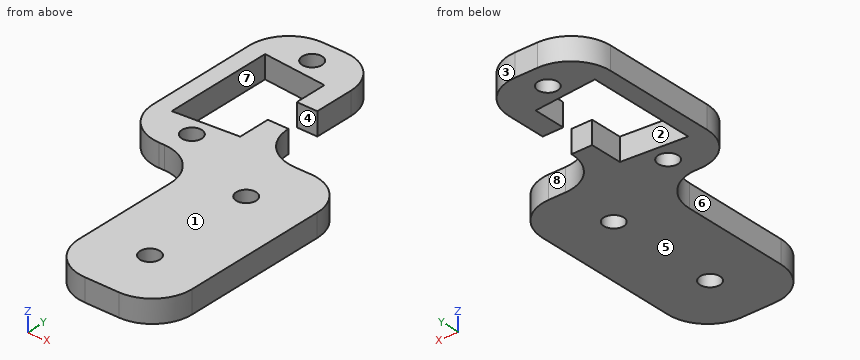
```python
from build123d import *

# Parameters (mm, degrees)
ESBO_O1_R                = 1.75
RESSALTO_EXTRUS_O1_DEPTH = 4
FILETE2_R                = 7


with BuildPart() as part:
    # Esboço1 → Ressalto-extrusão1 (new body)
    with BuildSketch(Plane.XY):
        Polygon((-9, -17), (6, -17), (6, -50), (26, -50), (26, -10), (9, -10), (9, -3), (5.359078591, -3), (5.359078591, -8.75), (-5.940921409, -9.7), (-5.940921409, 9.7), (5.359078591, 8.75), (5.359078591, 3), (9, 3), (9, 17), (-9, 17), align=None)
        with Locations((16, -40)):
            Circle(ESBO_O1_R, mode=Mode.SUBTRACT)
        with Locations((16, -20)):
            Circle(ESBO_O1_R, mode=Mode.SUBTRACT)
        with Locations((0, -12.5)):
            Circle(ESBO_O1_R, mode=Mode.SUBTRACT)
        with Locations((0, 12.5)):
            Circle(ESBO_O1_R, mode=Mode.SUBTRACT)
    extrude(amount=RESSALTO_EXTRUS_O1_DEPTH)

    # Filete2
    filete2_edges = [part.edges().sort_by_distance(p)[0] for p in [
        (6, -50, 2),
        (6, -17, 2),
        (-9, -17, 2),
        (-9, 17, 2),
        (9, 17, 2),
        (9, -10, 2),
        (26, -10, 2),
        (26, -50, 2),
    ]]
    fillet(filete2_edges, radius=FILETE2_R - 0.0001)  # a hair under: the kernel refuses the full size


solid = part.part
```
Work out the finished part from the listing and answer in its coordinate system (mm). Face numbers are marked on the shaded views. A direction names the side the tool comes from. Round coordinates to 2 decimals unless told otherwise and drop trailing zeros. Write each loop counter-clockwise with the first axis right and the second up, starting at its lowest first coordinate (ties: lowest second). Pieces come first, ordered by that corner, then holes. Notation, with made-up numbers: (-13, 16.5) -> (-6, 16.5) arc R27 cw to (-6, 38.5) -> close; hole circle Ø10 at (1, -13.5). An arc over 180 degrees is marked (long way). Write each question's results on one line, items separated by ' | '.
Q1. Flat-ended cylindrical pins translate along their axes: P1, Ø1.8, axis at x = 7.5, z = 1, coming from the +Y side; P2, Ø1.1, axis at x = 7.5, z = 1.5, coming from the -Y side. Find the tip coordinate at first contact, or state that the pin passes through.
Data:
P1: y = 15.28 | P2: y = -47.95
Q2. Determine the mould class of the marked faces 1, 2 and 3 for opening direction X: released by +X, released by -X, zero draft, split by the parting line, or undercut.
Data:
face 1: zero draft | face 2: undercut | face 3: released by +X
Q3. Which of the six approach directions +Z, -Z, +X, -X, +Y, -Y give full straight-line access (tool end or side, diameter ignored) to the marked faces 4, 5, 6, 7 and 8?
Data:
face 4: +Z, -Z, +X | face 5: -Z, +X, -X, +Y, -Y | face 6: +Z, -Z, -X, -Y | face 7: +Z, -Z | face 8: +Z, -Z, +X, +Y
Q4. Section C-C, the plane x = 3.5 is taken. Write down the section's boundary in (y, z), then the cut area to 3 significant figures.
Data:
outline: (-18.64, 0) -> (-8.91, 0) -> (-8.91, 4) -> (-18.64, 4) -> close; (8.91, 0) -> (16.84, 0) -> (16.84, 4) -> (8.91, 4) -> close | area: 70.7 mm^2
Q5. Section D-D, the plane x = 15 is taken. Write down the section's boundary in (y, z).
Data:
outline: (-50, 0) -> (-41.44, 0) -> (-41.44, 4) -> (-50, 4) -> close; (-38.56, 0) -> (-21.44, 0) -> (-21.44, 4) -> (-38.56, 4) -> close; (-18.56, 0) -> (-9.93, 0) -> (-9.93, 4) -> (-18.56, 4) -> close
Q6. Straight lines are drawn through the part: line 1 along Y through (x, z) = (16, 1.4); line 2 along Y through (x, z) = (0, 2.65); line 3 along Y through (x, z) = (-0.5, 1.7). For each, find the intervals that lie inside material, in ascending order. Write a range as [from, to].
Data:
line 1: [-50, -41.75], [-38.25, -21.75], [-18.25, -10] | line 2: [-17.07, -14.25], [-10.75, -9.2], [9.2, 10.75], [14.25, 17] | line 3: [-17.02, -14.18], [-10.82, -9.24], [9.24, 10.82], [14.18, 17]
Q7. Section B-B, the plane z = 3.25 is taken. Give the number of separate pieces and of enclosed holes in the cut face, then the cut area to 3 significant figures.
Data:
separate pieces: 1 | enclosed holes: 4 | area: 1,080 mm^2
Q8. Section A-A, the plane y = -40 is taken. Write down the section's boundary in (x, z), then the cut area to 3 significant figures.
Data:
outline: (6, 0) -> (14.25, 0) -> (14.25, 4) -> (6, 4) -> close; (17.75, 0) -> (26, 0) -> (26, 4) -> (17.75, 4) -> close | area: 66.0 mm^2
